Source: CAD feature listing. Evaluate the final solid. Frame: model axes, mm. Face numbers are marked on the shaded views. Round coordinates to 2 decimals unless told otherwise and drop trailing zeros. Order: outer loops, then holes, each group sorted by start corner. A loop starts at its lowest first (then second) coordinate and runs counter-clockwise, first axis right, second up. Notation, with made-up numbers: (-28.5, -13.75) - (0.5, -13.75) arc R11 ccw to (0.5, 3.25) - close; hole circle Ø10 at (6, -39). An arc over 180 degrees is marked (long way). Use one line per item in the form item = value. Start each with the question number.
Q1. Draft query along Y for the marked faces 1, 2 and 3. Return one class per face: released by +Y, released by -Y, zero draft, split by the parting line, or undercut.
Q2. Cut plane B-B, the plane z = 1.5. Give the number of separate pieces and of enclosed holes in the cut face, and give its area (3 significant figures).
Q3. Cut plane C-C, the plane x = 232. Return the cut outline in (y, z).
Q4. Pin query (flat end, axial travel): pin 1 Ø3 at (y, z) = (305, 2) entering from -X; pin 2 Ø1.4 at (y, z) = (323.5, 2.5) entering from +X; pin 3 Ø2.5 at (y, z) = (324, 5) entering from -X. Return the tip coordinate at first contact, or that it passes through.
Q5. Cut plane A-A, the plane y = 249.5. Return the cut outline in (x, z), and give its area (3 significant figures).
Q6. Ray query, line 1 (X direction, y = 253, z = 6); line 2 (X direction, y = 246.5, z = 4.25); line 3 (X direction, y = 270.5, z = 4.5). Return the intervals inside material, ascending. Write a range as [from, to].
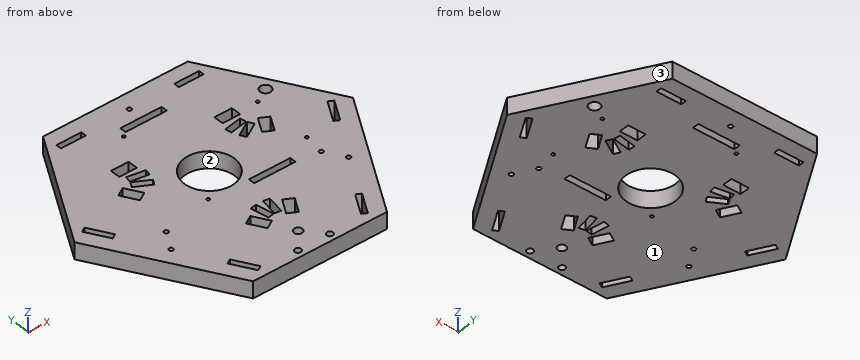
from build123d import *

# Parameters (mm, degrees)
ESBO_O2_R                = 2
ESBO_O2_R_2              = 1.5
ESBO_O2_R_3              = 1
ESBO_O2_R_4              = 0.75
ESBO_O2_R_5              = 2.6
ESBO_O2_R_6              = 12
ESBO_O2_W                = 12
ESBO_O2_H                = 2.6
ESBO_O2_W_2              = 8.5
ESBO_O2_H_2              = 4.75
ESBO_O2_W_3              = 20
ESBO_O2_H_3              = 3
RESSALTO_EXTRUS_O1_DEPTH = 8


with BuildPart() as part:
    # Esboço2 → Ressalto-extrusão1 (new body)
    with BuildSketch(Plane.XY):
        Polygon((312.401923789, 240.878221735), (347.401923789, 301.5), (315, 357.621778265), (245, 357.621778265), (212.598076211, 301.5), (247.598076211, 240.878221735), align=None)
        with Locations((280, 253.378221735)):
            Circle(ESBO_O2_R, mode=Mode.SUBTRACT)
        with Locations((272.260343171, 244.388972359)):
            Circle(ESBO_O2_R_2, mode=Mode.SUBTRACT)
        with Locations((287.760343171, 244.388972359)):
            Circle(ESBO_O2_R_2, mode=Mode.SUBTRACT)
        with Locations((242.5, 284.378221735)):
            Circle(ESBO_O2_R_3, mode=Mode.SUBTRACT)
        with Locations((317.5, 284.378221735)):
            Circle(ESBO_O2_R_3, mode=Mode.SUBTRACT)
        with Locations((267.750492284, 338.382369461)):
            Circle(ESBO_O2_R_4, mode=Mode.SUBTRACT)
        with Locations((267, 289.378221735)):
            Circle(ESBO_O2_R_4, mode=Mode.SUBTRACT)
        with Locations((319, 294.378221735)):
            Circle(ESBO_O2_R_4, mode=Mode.SUBTRACT)
        with Locations((319, 322.378221735)):
            Circle(ESBO_O2_R_4, mode=Mode.SUBTRACT)
        with Locations((280, 349.621778265)):
            Circle(ESBO_O2_R_3, mode=Mode.SUBTRACT)
        with Locations((237.026279442, 275.189110868)):
            Circle(ESBO_O2_R_3, mode=Mode.SUBTRACT)
        with Locations((322.973720558, 275.189110868)):
            Circle(ESBO_O2_R_3, mode=Mode.SUBTRACT)
        with Locations((326.159646677, 326.362840761)):
            Circle(ESBO_O2_R_5, mode=Mode.SUBTRACT)
        with Locations((278.32399049, 302.032244112)):
            Circle(ESBO_O2_R_6, mode=Mode.SUBTRACT)
        with Locations((251.453146627, 349.186651246)):
            Rectangle(ESBO_O2_W, ESBO_O2_H, mode=Mode.SUBTRACT)
        with Locations((308.5, 349.259600438)):
            Rectangle(ESBO_O2_W, ESBO_O2_H, mode=Mode.SUBTRACT)
        Polygon((332.76851184, 295.516364843), (335.020177889, 294.216364843), (341.020177889, 304.608669688), (338.76851184, 305.908669688), align=None, mode=Mode.SUBTRACT)
        Polygon((310.272092192, 256.543153732), (312.523758242, 255.243153732), (306.520177889, 244.852916827), (304.26851184, 246.152916827), align=None, mode=Mode.SUBTRACT)
        Polygon((255.623234985, 246.090416827), (253.371568935, 244.790416827), (247.371568935, 255.182721672), (249.623234985, 256.482721672), align=None, mode=Mode.SUBTRACT)
        Polygon((227.123234985, 295.453864843), (224.871568935, 294.153864843), (218.871568935, 304.546169688), (221.123234985, 305.846169688), align=None, mode=Mode.SUBTRACT)
        with Locations((305, 323.246778265)):
            Rectangle(ESBO_O2_W_2, ESBO_O2_H_2, mode=Mode.SUBTRACT)
        Polygon((312.7004902, 314.895353928), (308.4504902, 307.534137996), (312.564110868, 305.159137996), (316.814110868, 312.520353928), align=None, mode=Mode.SUBTRACT)
        with Locations((255, 323.246778265)):
            Rectangle(ESBO_O2_W_2, ESBO_O2_H_2, mode=Mode.SUBTRACT)
        Polygon((251.5495098, 307.534137996), (247.2995098, 314.895353928), (243.185889132, 312.520353928), (247.435889132, 305.159137996), align=None, mode=Mode.SUBTRACT)
        Polygon((272.2995098, 271.594083739), (268.185889132, 269.219083739), (272.435889132, 261.857867807), (276.5495098, 264.232867807), align=None, mode=Mode.SUBTRACT)
        Polygon((287.7004902, 271.594083739), (283.4504902, 264.232867807), (287.564110868, 261.857867807), (291.814110868, 269.219083739), align=None, mode=Mode.SUBTRACT)
        Polygon((279.8, 267.1), (278.32399049, 275.470865901), (275.369567231, 274.949921368), (276.845576741, 266.579055467), align=None, mode=Mode.SUBTRACT)
        Polygon((281.67600951, 275.470865901), (280.2, 267.1), (283.154423259, 266.579055467), (284.630432769, 274.949921368), align=None, mode=Mode.SUBTRACT)
        Polygon((308.136808057, 315.624122952), (300.775592125, 311.374122952), (302.275592125, 308.77604674), (309.636808057, 313.02604674), align=None, mode=Mode.SUBTRACT)
        Polygon((299.629134099, 314.52399049), (308, 316), (307.479055467, 318.954423259), (299.108189566, 317.478413749), align=None, mode=Mode.SUBTRACT)
        Polygon((251.907080103, 316.160436254), (260.277946003, 314.684426744), (260.798890536, 317.638850003), (252.428024636, 319.114859513), align=None, mode=Mode.SUBTRACT)
        Polygon((259.131487977, 311.534559206), (251.770272045, 315.784559206), (250.270272045, 313.186482994), (257.631487977, 308.936482994), align=None, mode=Mode.SUBTRACT)
        with Locations((280, 341.5)):
            Rectangle(ESBO_O2_W_3, ESBO_O2_H_3, mode=Mode.SUBTRACT)
        with Locations((296.230303561, 287.270994592)):
            Rectangle(ESBO_O2_W_3, ESBO_O2_H_3, mode=Mode.SUBTRACT)
    extrude(amount=RESSALTO_EXTRUS_O1_DEPTH)


solid = part.part
Completed:
q1.face_1 = zero draft
q1.face_2 = undercut
q1.face_3 = released by +Y
q2.separate_pieces = 1
q2.enclosed_holes = 34
q2.area = 10,600 mm2
q3.outline = (267.89, 0) - (335.11, 0) - (335.11, 8) - (267.89, 8) - close
q4.pin_1 = 213.75
q4.pin_2 = 335.1
q4.pin_3 = 224.87
q5.outline = (242.62, 0) - (250.65, 0) - (250.65, 8) - (242.62, 8) - close; (253.65, 0) - (306.2, 0) - (306.2, 8) - (253.65, 8) - close; (309.21, 0) - (317.38, 0) - (317.38, 8) - (309.21, 8) - close
q5.area = 550 mm2
q6.line_1 = [240.6, 248.63], [251.63, 278.04], [281.96, 308.22], [311.23, 319.4]
q6.line_2 = [244.35, 252.38], [255.39, 304.47], [307.47, 315.65]
q6.line_3 = [230.5, 270.4], [272.93, 276.15], [279.2, 280.8], [283.85, 287.07], [289.6, 329.5]
